Input: part model. Units: mm. Frame: model coordinates. Face numbers are marked on the shaded views. Coordinates: 2 decimals unless noted, no trailing zeros. Order: outer loops, then holes, each group sorted by start corner. A loop starts at its lowest first (then second) coordinate and runs counter-clockwise, first axis right, second up.
from build123d import *

# Parameters (mm, degrees)
SKETCH1_W           = 5
SKETCH1_H           = 5
SKETCH1_W_2         = 2
SKETCH1_H_2         = 2
BOSS_EXTRUDE1_DEPTH = 2
SKETCH1_4_W         = 5
SKETCH1_4_H         = 5
BOSS_EXTRUDE2_DEPTH = 4
SKETCH1_5_W         = 2
SKETCH1_5_H         = 2
BOSS_EXTRUDE3_DEPTH = 6


with BuildPart() as part:
    # Sketch1 → Boss-Extrude1 (new body)
    # profile 1 of 7: a face of its own
    with BuildSketch(Plane(origin=(0, 0, 0), x_dir=(1, 0, 0), z_dir=(0, 1, 0))):
        Polygon((-1, 53), (-1, 51), (-3, 51), (-3, -3), (73, -3), (73, 53), align=None)
        Polygon((-1, 46), (-1, 51), (4, 51), (66, 51), (71, 51), (71, 46), (71, 4), (71, -1), (66, -1), (4, -1), (-1, -1), (-1, 4), align=None, mode=Mode.SUBTRACT)
    # profile 2 of 7: a face of its own
    with BuildSketch(Plane(origin=(0, 0, 0), x_dir=(1, 0, 0), z_dir=(0, 1, 0))):
        with Locations((68.5, 1.5)):
            Rectangle(SKETCH1_W, SKETCH1_H)
    # profile 3 of 7: a face of its own
    with BuildSketch(Plane(origin=(0, 0, 0), x_dir=(1, 0, 0), z_dir=(0, 1, 0))):
        Polygon((66, 51), (4, 51), (4, 46), (-1, 46), (-1, 4), (4, 4), (4, -1), (66, -1), (66, 4), (71, 4), (71, 46), (66, 46), align=None)
    # profile 4 of 7: a face of its own
    with BuildSketch(Plane(origin=(0, 0, 0), x_dir=(1, 0, 0), z_dir=(0, 1, 0))):
        with Locations((68.5, 48.5)):
            Rectangle(SKETCH1_W, SKETCH1_H)
    # profile 5 of 7: a face of its own
    with BuildSketch(Plane(origin=(0, 0, 0), x_dir=(1, 0, 0), z_dir=(0, 1, 0))):
        with Locations((1.5, 1.5)):
            Rectangle(SKETCH1_W, SKETCH1_H)
    # profile 6 of 7: a face of its own
    with BuildSketch(Plane(origin=(0, 0, 0), x_dir=(1, 0, 0), z_dir=(0, 1, 0))):
        with Locations((1.5, 48.5)):
            Rectangle(SKETCH1_W, SKETCH1_H)
    # profile 7 of 7: a face of its own
    with BuildSketch(Plane(origin=(0, 0, 0), x_dir=(1, 0, 0), z_dir=(0, 1, 0))):
        with Locations((-2, 52)):
            Rectangle(SKETCH1_W_2, SKETCH1_H_2)
    extrude(amount=BOSS_EXTRUDE1_DEPTH)

    # Sketch1_4 → Boss-Extrude2 (add)
    with BuildSketch(Plane(origin=(0, 0, 0), x_dir=(1, 0, 0), z_dir=(0, 1, 0))):
        with Locations((1.5, 1.5)):
            Rectangle(SKETCH1_4_W, SKETCH1_4_H)
        with Locations((1.5, 48.5)):
            Rectangle(SKETCH1_4_W, SKETCH1_4_H)
        with Locations((68.5, 48.5)):
            Rectangle(SKETCH1_4_W, SKETCH1_4_H)
        with Locations((68.5, 1.5)):
            Rectangle(SKETCH1_4_W, SKETCH1_4_H)
    extrude(amount=BOSS_EXTRUDE2_DEPTH)

    # Sketch1_5 → Boss-Extrude3 (add)
    # profile 1 of 2: a face of its own
    with BuildSketch(Plane(origin=(0, 0, 0), x_dir=(1, 0, 0), z_dir=(0, 1, 0))):
        Polygon((-1, 53), (-1, 51), (-3, 51), (-3, -3), (73, -3), (73, 53), align=None)
        Polygon((-1, 46), (-1, 51), (4, 51), (66, 51), (71, 51), (71, 46), (71, 4), (71, -1), (66, -1), (4, -1), (-1, -1), (-1, 4), align=None, mode=Mode.SUBTRACT)
    # profile 2 of 2: a face of its own
    with BuildSketch(Plane(origin=(0, 0, 0), x_dir=(1, 0, 0), z_dir=(0, 1, 0))):
        with Locations((-2, 52)):
            Rectangle(SKETCH1_5_W, SKETCH1_5_H)
    extrude(amount=BOSS_EXTRUDE3_DEPTH)


solid = part.part
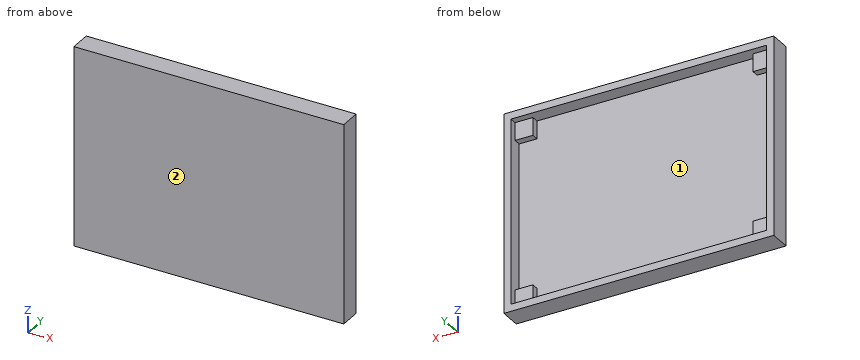
Item 1: Pin query (flat end, axial travel): pin 1 Ø4 at (x, z) = (68, -47.5) entering from +Y. Return the tip coordinate at first contact, or that it passes through.
Response values:
pin 1: stops at y = 4
Item 2: Cut plane D-D on x = 35. Return loops of the section in (y, z), then the cut area to 3 significant figures.
Response values:
outline: (0, -53) - (6, -53) - (6, -51) - (2, -51) - (2, 1) - (6, 1) - (6, 3) - (0, 3) - close
area: 128 mm2
Item 3: Ray query, probe 1 along Z at (x, y) = (42, 3.55); probe 2 along X at (y, z) = (5.55, -49.5); probe 3 along X at (y, z) = (3.4, -47). Return the intervals inside material, ascending.
Response values:
probe 1: z = -53 to -51, 1 to 3
probe 2: x = -3 to -1, 71 to 73
probe 3: x = -3 to 4, 66 to 73
Item 4: Draft query along Z for the marked faces 1 and 2. Return one class per face: pulls with the +Z half, pulls with the -Z half, needs draft (parallel to the pull), parting line crosses it, or undercut.
Response values:
face 1: undercut
face 2: needs draft
Item 5: Cut plane B-B on y = 3.05. Return loops of the section in (x, z).
Response values:
outline: (-3, -53) - (73, -53) - (73, 3) - (-3, 3) - close; hole (-1, -46) - (4, -46) - (4, -51) - (66, -51) - (66, -46) - (71, -46) - (71, -4) - (66, -4) - (66, 1) - (4, 1) - (4, -4) - (-1, -4) - close
Item 6: Cut plane A-A on x = 67. Return loops of the section in (y, z).
Response values:
outline: (0, -53) - (6, -53) - (6, -51) - (4, -51) - (4, -46) - (2, -46) - (2, -4) - (4, -4) - (4, 1) - (6, 1) - (6, 3) - (0, 3) - close
Item 7: Cut plane C-C on z = -13. Return loops of the section in (x, y).
Response values:
outline: (-3, 0) - (73, 0) - (73, 6) - (71, 6) - (71, 2) - (-1, 2) - (-1, 6) - (-3, 6) - close
